Geometry check sheet. Reference: the model listing, model coordinates, mm. Round coordinates to 2 decimals unless told otherwise and drop trailing zeros. Write each loop counter-clockwise with the first axis right and the second up, starting at its lowest first coordinate (ties: lowest second). Pieces come first, ordered by that corner, then holes. Notation, with made-up numbers: M 24,22.25 L 30,22.25 A15 cw 30,37.25 Z; hole C 69,76 d6. An arc over 180 degrees is marked long. One line per item, written item: value. Start each with the question number.
1. Section check A-A (x = 25). Record the boundary of the cut face in (y, z).
2. Scan lines: probe 1 along Y at (x, z) = (25.5, 0.6); probe 2 along X at (y, z) = (9.5, 0.75); probe 3 along X at (y, z) = (57.5, 0.85). Record each from-to range of solid material in increasing order. Write a range as [from, to].
3. Section check C-C (y = 53.75). Record the boundary of the cut face in (x, z), and give its area (3 significant figures).
4. Section check D-D (y = -2). Record the boundary of the cut face in (x, z), and give its area (3 significant figures).
5. Section check B-B (z = 0.6). Record the boundary of the cut face in (x, y).
6. Depth check by flat-ended pin: P1, Ø15.5, axis at x = 25, y = -2, coming from the -Z side; P2, Ø0.5, axis at y = 34, z = 0.5, coming from the +X side. Enter the tip coordinate at first touch or a pass-through.
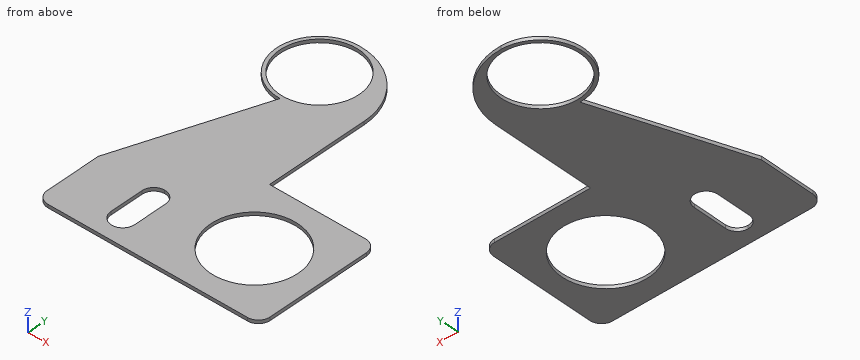
from build123d import *

# Parameters (mm, degrees)
F0_R     = 13
F0_R_2   = 11.75
F1_DEPTH = 1


with BuildPart() as f1:
    # F0 (on Top) → F1 (new body)
    with BuildSketch(Plane.XY):
        with BuildLine():
            ThreePointArc((-7, 66.5), (2.015611, 62.765611), (5.75, 53.75))
            ThreePointArc((5.75, 53.75), (2.015611, 44.734389), (-7, 41))
            Line((-7, 41), (-22.28675, -1))
            Line((-22.28675, -1), (-22.28675, -17.5))
            ThreePointArc((-22.28675, -17.5), (-21.261624, -19.974874), (-18.78675, -21))
            Line((-18.78675, -21), (40.5, -21))
            ThreePointArc((40.5, -21), (42.974874, -19.974874), (44, -17.5))
            Line((44, -17.5), (44, 13.5))
            ThreePointArc((44, 13.5), (42.974874, 15.974874), (40.5, 17))
            Line((40.5, 17), (12, 17))
            Line((12, 17), (12, 47.5))
            ThreePointArc((12, 47.5), (6.435029, 60.935029), (-7, 66.5))
        make_face()
        with BuildLine():
            ThreePointArc((-3.5, 0), (-1.025126, -1.025126), (0, -3.5))
            Line((0, -3.5), (0, -13.5))
            ThreePointArc((0, -13.5), (-1.025126, -15.974874), (-3.5, -17))
            ThreePointArc((-3.5, -17), (-5.974874, -15.974874), (-7, -13.5))
            Line((-7, -13.5), (-7, -3.5))
            ThreePointArc((-7, -3.5), (-5.974874, -1.025126), (-3.5, 0))
        make_face(mode=Mode.SUBTRACT)
        with Locations((25, -2)):
            Circle(F0_R, mode=Mode.SUBTRACT)
        with BuildLine():
            ThreePointArc((-7, 41), (2.015611, 44.734389), (5.75, 53.75))
            ThreePointArc((5.75, 53.75), (2.015611, 62.765611), (-7, 66.5))
            ThreePointArc((-7, 66.5), (-19.75, 53.75), (-7, 41))
        make_face()
        with Locations((-7, 53.75)):
            Circle(F0_R_2, mode=Mode.SUBTRACT)
    extrude(amount=F1_DEPTH)


solid = f1.part
Result sheet:
1. outline: M -21,0 L -15,0 L -15,1 L -21,1 Z; M 11,0 L 17,0 L 17,1 L 11,1 Z
2. probe 1: y = [-21, -14.99], [10.99, 17]
2. probe 2: x = [-18.47, 18.94], [31.06, 44]
2. probe 3: x = [-19.19, -18.14], [4.14, 9.16]
3. outline: M -19.75,0 L -18.75,0 L -18.75,1 L -19.75,1 Z; M 4.75,0 L 10.94,0 L 10.94,1 L 4.75,1 Z
3. area: 7.19 mm2
4. outline: M -22.29,0 L -6.66,0 L -6.66,1 L -22.29,1 Z; M -0.34,0 L 12,0 L 12,1 L -0.34,1 Z; M 38,0 L 44,0 L 44,1 L 38,1 Z
4. area: 34.0 mm2
5. outline: M -22.29,-17.5 A3.5 ccw -18.79,-21 L 40.5,-21 A3.5 ccw 44,-17.5 L 44,13.5 A3.5 ccw 40.5,17 L 12,17 L 12,47.5 A19 ccw -7,66.5 A12.75 ccw -7,41 L -22.29,-1 Z; hole C -7,53.75 d23.5; hole M -7,-13.5 A3.5 ccw -3.5,-17 A3.5 ccw 0,-13.5 L 0,-3.5 A3.5 ccw -3.5,0 A3.5 ccw -7,-3.5 Z; hole C 25,-2 d26
6. P1: passes through
6. P2: stops at x = 12
